The model under review builds one solid part; all positions refer to its coordinate system, in mm. Coordinates: 2 decimals unless noted, no trailing zeros. Write each loop counter-clockwise with the first axis right and the second up, starting at its lowest first coordinate (ties: lowest second). Pieces come first, ordered by that corner, then holes. Notation, with made-up numbers: (-17, 74.25) - (24, 74.25) arc R21 cw to (24, 98.25) - close; hole circle Ø9 at (3, -34.5). An arc over 180 degrees is marked (long way). Answer as CSV lines item,"result". Start each with the question number.
Autodesk Inventor part; units mm, degrees
ref_plane "YZ Plane" through (0, 0, 0) normal (1, 0, 0) x (0, 1, 0)
ref_plane "XZ Plane" through (0, 0, 0) normal (0, 1, 0) x (-1, 0, 0)
ref_plane "XY Plane" through (0, 0, 0) normal (0, 0, 1) x (1, 0, 0)
sketch "Sketch1" plane through (0, 0, 0) normal (0, 1, 0) x (-1, 0, 0)
  line L0 (13.325, 0) -> (-13.325, 0) construction
  line L1 (13.325, 10) -> (-13.325, 10)
  line L2 (-13.325, -10) -> (13.325, -10)
  arc A0 (13.325, -10) -> (13.325, 10) centre (13.325, 0) ccw
  arc A1 (-13.325, 10) -> (-13.325, -10) centre (-13.325, 0) ccw
  point P0 (0, 0)
  dimension "d0" = 26.65
  dimension "d1" = 20
extrude "Extrusion1" add sketch "Sketch1" along normal blind 3
sketch "Sketch2" plane through (0, 3, 0) normal (0, 1, 0) x (1, 0, 0)
  point P0 (0, 0)
  point P1 (-17.33, 0)
  point P2 (-4.33, 0)
  dimension "d4" = 17.33
  dimension "d5" = 4.33
hole "Hole1" at (-17.33, 3, 0) at (-4.33, 3, 0) direction (0, -1, 0) diameter 4.2 end through all
sketch "Sketch3" plane through (0, 3, 0) normal (0, 1, 0) x (1, 0, 0)
  line L0 (-32.655, 0) -> (32.655, 0)
  point P0 (0, 0)
  point P1 (11.68, 1)
  dimension "d13" = 1
  dimension "d14" = 11.68
hole "Hole2" at (11.68, 3, -1) direction (0, -1, 0) diameter 8.2 end through all
properties part number "X Adjustment Block" material "Aluminum 6061"
(1) Add section A-A on x = -4.33. Give the boundary of the cut face in (y, z), then the cut area to 3 significant figures.
(2) Wall thickness on line 1 (Z direction, x = -4.5, y = 2.75); line 2 (X direction, y = 1.35, z = 0) (3 decimals); line 3 (Z direction, x = 11.68, y = 2.3): over which ranges is each line inside the solid? List them lowest first.
(3) Add section B-B on y = 0.8. Give the boundary of the cut face in (x, z) (3 decimals), then the cut area to 3 significant figures.
(4) Add section D-D on x = 10. Give the boundary of the cut face in (y, z).
(5) The part is to be moulded in two halves that separate along Z. For faces 1 (the cylindrical face through (10.45, 1.48, 2.91)), 2 (the cylindrical face through (-2.467, 1.479, 0.969)), 3 (the flat face through (0, 3, 0)), 4 (the cylindrical face through (23.323, 1.479, -0.22)), say which applies: released by +Z, released by -Z, zero draft, split by the parting line, or undercut.
(6) For pin 1 (4 mm diameter, centred on x = -17.33, z = 0, fed in from +Y); pin 2 (1 mm diameter, centred on y = 1, z = -6, fed in from -X), all flat-tipped, find the tip position at first contact; note any pin that passes through.
(7) Add section C-C on z = -1. Give the boundary of the cut face in (x, y).
Reported:
1,outline,"(0, -10) - (3, -10) - (3, -2.1) - (0, -2.1) - close; (0, 2.1) - (3, 2.1) - (3, 10) - (0, 10) - close"
1,area,"47.4 mm²"
2,line 1,"-10 to -2.09, 2.09 to 10"
2,line 2,"-23.325 to -19.43, -15.23 to -6.43, -2.23 to 7.704, 15.656 to 23.325"
2,line 3,"-10 to -5.1, 3.1 to 10"
3,outline,"(-13.325, -10) - (13.325, -10) arc R10 ccw to (13.325, 10) - (-13.325, 10) arc R10 ccw to start; hole circle Ø4.2 at (-17.33, 0); hole circle Ø4.2 at (-4.33, 0); hole circle Ø8.2 at (11.68, -1)"
3,area,"767 mm²"
4,outline,"(0, -10) - (3, -10) - (3, -4.74) - (0, -4.74) - close; (0, 2.74) - (3, 2.74) - (3, 10) - (0, 10) - close"
5,face 1,"undercut"
5,face 2,"undercut"
5,face 3,"zero draft"
5,face 4,"split by the parting line"
6,pin 1,"through"
6,pin 2,"x = -21.68"
7,outline,"(-23.27, 0) - (-19.18, 0) - (-19.18, 3) - (-23.27, 3) - close; (-15.48, 0) - (-6.18, 0) - (-6.18, 3) - (-15.48, 3) - close; (-2.48, 0) - (7.58, 0) - (7.58, 3) - (-2.48, 3) - close; (15.78, 0) - (23.27, 0) - (23.27, 3) - (15.78, 3) - close"
